Geometry: final body of the model. Coordinates: model frame, mm. Face numbers are marked on the shaded views. A direction names the side the tool comes from. Coordinates: 2 decimals unless noted, no trailing zeros. Order: outer loops, then holes, each group sorted by start corner. A loop starts at its lowest first (then second) coordinate and runs counter-clockwise, first axis right, second up. Notation, with made-up numbers: M 17,29 L 57,29 A15 cw 57,50 Z; hole C -35.75,-24.75 d4. An arc over 180 degrees is marked long. One line per question, with ' | ' between items.
from build123d import *

# Parameters (mm, degrees)
F1_DEPTH  = 200
F4_DEPTH  = 110
F5_W      = 20
F5_H      = 50
F6_DEPTH  = 110
F7_R      = 10
F7_R_2    = 9.99999
F8_R      = 10
F12_DEPTH = 100


# Not quite as in the source:
# - a fillet or chamfer is up to 0.001 mm smaller than in the source, because OpenCascade refuses the exact size


with BuildPart() as f1:
    # F0 (on Top) → F1 (new body)
    with BuildSketch(Plane.XY):
        with BuildLine():
            Line((-129.7011448747, 82.0831308431), (-195, 55.2543373544))
            Line((-195, 55.2543373544), (-195, 0.2543373544))
            Line((-195, 0.2543373544), (195, 0.2543373544))
            Line((195, 0.2543373544), (195, 20.2543373544))
            ThreePointArc((195, 20.2543373544), (178.031605372, 64.0489133357), (135.9856958342, 84.9781463073))
            Line((135.9856958342, 84.9781463073), (-16.3916033039, 99.0700883522))
            ThreePointArc((-16.3916033039, 99.0700883522), (-74.0749348766, 97.4375057422), (-129.7011448747, 82.0831308431))
        make_face()
        with BuildLine():
            Line((195, 0.2543373544), (-195, 0.2543373544))
            Line((-195, 0.2543373544), (-195, -54.7456626456))
            Line((-195, -54.7456626456), (-129.7011448747, -81.5744561343))
            ThreePointArc((-129.7011448747, -81.5744561343), (-74.0749348766, -96.9288310334), (-16.3916033039, -98.5614136434))
            Line((-16.3916033039, -98.5614136434), (135.9856958342, -84.4694715986))
            ThreePointArc((135.9856958342, -84.4694715986), (178.031605372, -63.540238627), (195, -19.7456626456))
            Line((195, -19.7456626456), (195, 0.2543373544))
        make_face()
    extrude(amount=F1_DEPTH)

    # F3 (on Front) → F4 (cut, symmetric)
    with BuildSketch(Plane.XZ):
        Polygon((195, 200), (-195, 200), (-195, 153), align=None)
    extrude(amount=F4_DEPTH, both=True, mode=Mode.SUBTRACT)

    # F5 (on Front) → F6 (cut, symmetric)
    with BuildSketch(Plane.XZ):
        with Locations((-35, 25)):
            Rectangle(F5_W, F5_H)
    extrude(amount=F6_DEPTH, both=True, mode=Mode.SUBTRACT)

    # F7 (call 1 of 2: OpenCascade refuses the feature's edges together)
    f7_edges = [f1.edges().sort_by_distance(p)[0] for p in [
        (-25, 0.254337, 50),
    ]]
    fillet(f7_edges, radius=F7_R)

    # F7#2 (call 2 of 2) (radius 10 in the source; OpenCascade refuses exactly that, so slightly less here)
    f7_2_edges = [f1.edges().sort_by_distance(p)[0] for p in [
        (-45, 0.254337, 50),
    ]]
    fillet(f7_2_edges, radius=F7_R_2)

    # F8
    f8_edges = [f1.edges().sort_by_distance(p)[0] for p in [
        (-45, 0.254337, 0),
        (-25, 0.254337, 0),
    ]]
    fillet(f8_edges, radius=F8_R)

    # F9 (on offset) → F10 (join, up to the next surface of F1)
    with BuildSketch(Plane.XY.offset(220)):
        with BuildLine():
            Line((-105, -86.0161099703), (-105, 86.5247846791))
            ThreePointArc((-105, 86.5247846791), (-116.6965219134, 82.7558804952), (-128.181003028, 78.3832431737))
            Line((-128.181003028, 78.3832431737), (-191, 52.5733282266))
            Line((-191, 52.5733282266), (-191, -52.0646535178))
            Line((-191, -52.0646535178), (-128.181003028, -77.8745684649))
            ThreePointArc((-128.181003028, -77.8745684649), (-116.6965219134, -82.2472057865), (-105, -86.0161099703))
        make_face()
    extrude(until=Until.NEXT, dir=(0, 0, -1))

    # F11 (on Front) → F12 (cut, symmetric)
    with BuildSketch(Plane.XZ):
        Polygon((-191, 156.5037577633), (-105, 216.8246032937), (-105, 220), (-191, 220), align=None)
    extrude(amount=F12_DEPTH, both=True, mode=Mode.SUBTRACT)


solid = f1.part
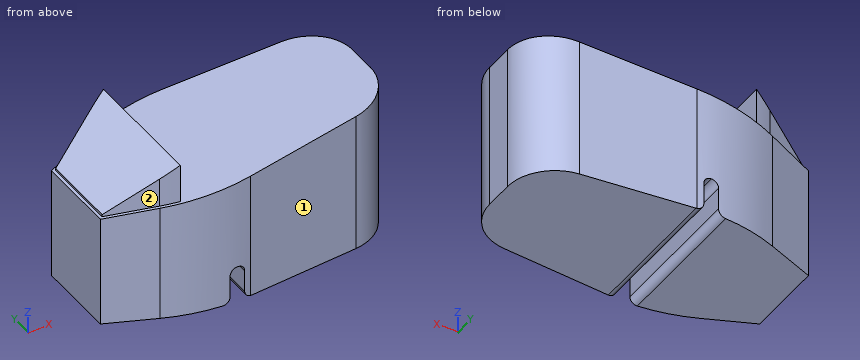
1. Pin query (flat end, axial travel): P1, Ø4, axis at x = -39.5, y = -70.5, coming from the -Z side; P2, Ø1.5, axis at y = -7, z = 155, coming from the -X side; P3, Ø10, axis at y = -38.5, z = 174, coming from the +X side. Return the tip coordinate at first contact, or that it passes through.
Response values:
P1: stops at z = 47.6 | P2: stops at x = -191 | P3: stops at x = 193.53
2. Access query for the marked faces 1 and 2. Directions: +Z, -Z, +X, -X, +Y, -Y. A direction counts if a zero-diameter tool reaches every point of the face in a straight line with its end or side. Return the directions, or none.
Response values:
face 1: +Z, -Z, +X, -Y | face 2: +Z, -X, -Y
3. Section C-C, the plane x = 71. Output: boundary loops of the cut face in (y, z).
Response values:
outline: M -90.48,0 L 90.99,0 L 90.99,185.06 L -90.48,185.06 Z
4. Section B-B, the plane z = 79.5. Output: boundary loops of the cut face in (x, y).
Response values:
outline: M -195,-54.75 L -129.7,-81.57 A240 ccw -16.39,-98.56 L 135.99,-84.47 A65 ccw 195,-19.75 L 195,20.25 A65 ccw 135.99,84.98 L -16.39,99.07 A240 ccw -129.7,82.08 L -195,55.25 Z
5. Material intervals for line 1 (X direction, y = 28.5, z = 32); line 2 (X direction, y = 53.5, z = 11.5); line 3 (Z direction, x = -11.5, y = -92), sorted ascending. Write a range as [from, to].
Response values:
line 1: x = [-195, -45], [-25, 194.47] | line 2: x = [-195, -45], [-25, 185.85] | line 3: z = [0, 175.11]
